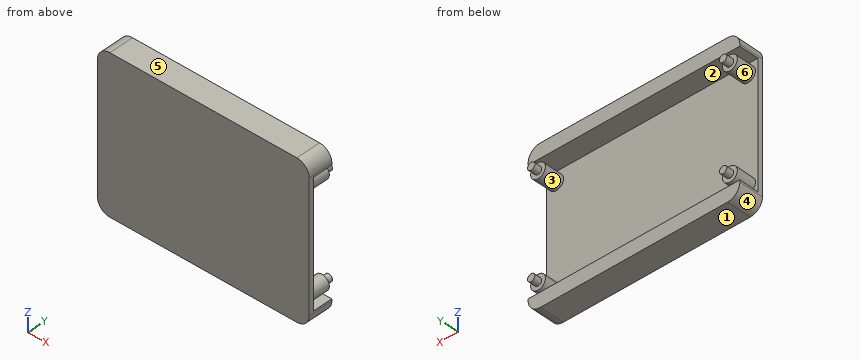
from build123d import *

# Parameters (mm, degrees)
SKETCH_1_W          = 86
SKETCH_1_H          = 62
EXTRUDE_1_DEPTH     = 10
SKETCH_2_W          = 86
SKETCH_2_H          = 50.4
SKETCH_2_R          = 3
CUT_EXTRUDE_1_DEPTH = 8
SKETCH_3_R          = 1.5
EXTRUDE_2_DEPTH     = 3
FILLET_1_R          = 5


with BuildPart() as part:
    # 草图1 → 凸台-拉伸1 (new body)
    with BuildSketch(Plane(origin=(0, 0, 0), x_dir=(1, 0, 0), z_dir=(0, 1, 0))):
        Rectangle(SKETCH_1_W, SKETCH_1_H)
    extrude(amount=EXTRUDE_1_DEPTH)

    # 草图2 → 切除-拉伸1 (cut)
    with BuildSketch(Plane(origin=(0, 10, 0), x_dir=(1, 0, 0), z_dir=(0, 1, 0))):
        Rectangle(SKETCH_2_W, SKETCH_2_H)
        with Locations(Location((-39, 21, 0), (0, 0, 270))):
            Circle(SKETCH_2_R, mode=Mode.SUBTRACT)
        with Locations(Location((39, 21, 0), (0, 0, 270))):
            Circle(SKETCH_2_R, mode=Mode.SUBTRACT)
        with Locations(Location((39, -21, 0), (0, 0, 270))):
            Circle(SKETCH_2_R, mode=Mode.SUBTRACT)
        with Locations(Location((-39, -21, 0), (0, 0, 270))):
            Circle(SKETCH_2_R, mode=Mode.SUBTRACT)
    extrude(amount=-CUT_EXTRUDE_1_DEPTH, mode=Mode.SUBTRACT)

    # 草图3 → 凸台-拉伸2 (add)
    with BuildSketch(Plane(origin=(0, 10, 0), x_dir=(1, 0, 0), z_dir=(0, 1, 0))):
        with Locations(Location((-39, 21, 0), (0, 0, 270))):
            Circle(SKETCH_3_R)
        with Locations(Location((39, 21, 0), (0, 0, 270))):
            Circle(SKETCH_3_R)
        with Locations(Location((39, -21, 0), (0, 0, 270))):
            Circle(SKETCH_3_R)
        with Locations(Location((-39, -21, 0), (0, 0, 270))):
            Circle(SKETCH_3_R)
    extrude(amount=EXTRUDE_2_DEPTH)

    # 圆角1
    fillet_1_edges = [part.edges().sort_by_distance(p)[0] for p in [
        (-43, 5, -31),
        (43, 5, -31),
        (43, 5, 31),
        (-43, 5, 31),
    ]]
    fillet(fillet_1_edges, radius=FILLET_1_R)


solid = part.part
Verification items for the finished model (mm, model axes). Face numbers are marked on the shaded views. A direction names the side the tool comes from. Coordinates: 2 decimals unless noted, no trailing zeros. Order: outer loops, then holes, each group sorted by start corner. A loop starts at its lowest first (then second) coordinate and runs counter-clockwise, first axis right, second up.
Item 1: Depth check by flat-ended pin: pin 1 (6 mm diameter, centred on x = 26, z = 0, fed in from +Y); pin 2 (4.5 mm diameter, centred on x = -17, z = -27, fed in from +Y). Enter the tip coordinate at first touch or a pass-through.
Filled in:
pin 1: stops at y = 2
pin 2: stops at y = 10
Item 2: Access from +Z, -Z, +X, -X, +Y, -Y to the whole of each face (thin tool, end or side, straight path). Record for the marked faces 1, 2 and 3.
Filled in:
face 1: -Z, +X, -X, +Y, -Y
face 2: +X, -X, +Y
face 3: +Y
Item 3: Section check C-C, the plane x = 17. Enter the section's corners in (y, z).
Filled in:
outline: (0, -31) - (10, -31) - (10, -25.2) - (2, -25.2) - (2, 25.2) - (10, 25.2) - (10, 31) - (0, 31) - close
Item 4: Section check B-B, the plane y = 7.75. Enter the section's corners in (x, z), then the cut area to 3 significant figures.
Filled in:
outline: (-43, -26) arc R5 ccw to (-38, -31) - (38, -31) arc R5 ccw to (43, -26) - (43, -25.2) - (-43, -25.2) - close; (-43, 25.2) - (43, 25.2) - (43, 26) arc R5 ccw to (38, 31) - (-38, 31) arc R5 ccw to (-43, 26) - close; circle Ø6 at (-39, -21); circle Ø6 at (-39, 21); circle Ø6 at (39, -21); circle Ø6 at (39, 21)
area: 1,090 mm2
Item 5: Release check for a two-part mould opening along X. For the marked faces 4, 5 and 6 record: +X half, -X half, draft (parallel to the pull), parting line (faces both ways), or undercut.
Filled in:
face 4: -X half
face 5: draft
face 6: undercut
Item 6: Section check D-D, the plane x = 39. Enter the section's corners in (y, z), then the cut area to 3 significant figures.
Filled in:
outline: (0, -30.9) - (10, -30.9) - (10, -25.2) - (2, -25.2) - (2, -24) - (10, -24) - (10, -22.5) - (13, -22.5) - (13, -19.5) - (10, -19.5) - (10, -18) - (2, -18) - (2, 18) - (10, 18) - (10, 19.5) - (13, 19.5) - (13, 22.5) - (10, 22.5) - (10, 24) - (2, 24) - (2, 25.2) - (10, 25.2) - (10, 30.9) - (0, 30.9) - close
area: 329 mm2
Item 7: Material ranges on L1, parallel to Z at x = 24, y = 4; L2, parallel to Y at x = -24, z = 0.5; L3, parallel to X at y = 5, z = 23.5, recorded low to high.
Filled in:
L1: z = -31 to -25.2, 25.2 to 31
L2: y = 0 to 2
L3: x = -40.66 to -37.34, 37.34 to 40.66
Item 8: Section check A-A, the plane z = 21. Enter the section's corners in (x, y), then the cut area to 3 significant figures.
Filled in:
outline: (-43, 0) - (43, 0) - (43, 2) - (42, 2) - (42, 10) - (40.5, 10) - (40.5, 13) - (37.5, 13) - (37.5, 10) - (36, 10) - (36, 2) - (-36, 2) - (-36, 10) - (-37.5, 10) - (-37.5, 13) - (-40.5, 13) - (-40.5, 10) - (-42, 10) - (-42, 2) - (-43, 2) - close
area: 286 mm2
